Model file for the job. Use its own axes, mm. A direction names the side the tool comes from. Give positions to 0.01 mm unless a question says otherwise; leave off trailing zeros. Order: outer loops, then holes, each group sorted by start corner. A loop starts at its lowest first (then second) coordinate and runs counter-clockwise, first axis right, second up. Notation, with made-up numbers: (40.25, 44.25) - (90.25, 44.25) arc R28 cw to (90.25, 83.25) - close; hole circle Ø3 at (81.5, 77.25). An arc over 180 degrees is marked (long way). Return JSON: item names as keys, results as strings. Group by question number.
Autodesk Inventor part; units mm, degrees
ref_plane "YZ Plane" through (0, 0, 0) normal (1, 0, 0) x (0, 1, 0)
ref_plane "XZ Plane" through (0, 0, 0) normal (0, 1, 0) x (-1, 0, 0)
ref_plane "XY Plane" through (0, 0, 0) normal (0, 0, 1) x (1, 0, 0)
sketch "Sketch1" plane through (0, 0, 0) normal (0, 0, 1) x (1, 0, 0)
  circle A0 centre (157.7925, 25.2801) radius 7.5
  circle A1 centre (157.7925, 25.2801) radius 4.05
  circle A2 centre (157.7925, -42.1199) radius 7.5
  circle A3 centre (157.7925, -42.1199) radius 4.05
  line L0 (7.5, 7.5) -> (-7.5, 7.5)
  line L1 (-7.5, 7.5) -> (-7.5, -74.9)
  line L2 (-7.5, -74.9) -> (7.5, -74.9)
  line L3 (7.5, -74.9) -> (7.5, 7.5)
  line L4 (7.5, 7.5) -> (-7.5, 7.5)
  line L5 (-7.5, 7.5) -> (-7.5, -74.9)
  line L6 (-7.5, -74.9) -> (7.5, -74.9)
  line L7 (7.5, -74.9) -> (7.5, 7.5)
  circle A4 centre (157.7925, 25.2801) radius 4.05
  circle A5 centre (157.7925, 25.2801) radius 7.5
  circle A6 centre (157.7925, 25.2801) radius 4.05
  circle A7 centre (157.7925, -42.1199) radius 4.05
  circle A8 centre (157.7925, -42.1199) radius 7.5
  circle A9 centre (157.7925, -42.1199) radius 4.05
  line L8 (7.5, 7.5) -> (-7.5, 7.5)
  line L9 (-7.5, 7.5) -> (-7.5, -74.9)
  line L10 (-7.5, -74.9) -> (7.5, -74.9)
  line L11 (7.5, -74.9) -> (7.5, 7.5)
  point P0 (0, 0)
extrude "Extrusion1" add sketch "Sketch1" against normal blind 10 contours A0 | A2
sketch "Sketch2" plane through (157.7925, 25.2801, 0) normal (0, 0, 1) x (1, 0, 0)
  line L0 (7.5, 7.5) -> (-7.5, 7.5)
  line L1 (-7.5, 7.5) -> (-7.5, -74.9)
  line L2 (-7.5, -74.9) -> (7.5, -74.9)
  line L3 (7.5, -74.9) -> (7.5, 7.5)
  circle A0 centre (0, 0) radius 7.5
  circle A1 centre (0, 0) radius 4.05
  circle A2 centre (0, -67.4) radius 7.5
  circle A3 centre (0, -67.4) radius 4.05
  circle A4 centre (0, -33.7) radius 7.5
  circle A5 centre (0, -33.7) radius 5
  point P0 (-157.7925, -25.2801)
  point P1 (7.5, 0)
  point P2 (-7.5, 0)
  point P3 (-7.5, -67.4)
  point P4 (7.5, -67.4)
  dimension "d2" = 10
extrude "Extrusion2" add sketch "Sketch2" along normal blind 10 contours L3 A0 L0 | A0 L1 L0 | A0 | L3 A4 L1 A0 | A4 | L3 A2 L1 A4 | A2 | L3 L2 A2 | A2 L2 L1 | A1 | A3
fillet "Fillet1" radius 2 4 edges at (150.2925, -49.6199, 5) (165.2925, -49.6199, 5) (165.2925, 32.7801, 5) (150.2925, 32.7801, 5)
properties part number "constraining plate"
(1) Drop a flat-ended pin along its axis: pin 1 Ø1.5 at (x, y) = (155, 4) entering from -Z. Give the stop position or say it passes through.
(2) Slice it at A-A (z = -6.25). Give the cut face in (x, y).
(3) 3-axis set-ups, long thin cutter, end or side, ignore diameter. For faces 4 (the face through (158, 25, 0)), 5 (the face through (164.7, 32.2, 5.1)), 6 (the face through (152, -48, 0)): which of +Z, -Z, +X, -X, +Y, -Y reach the whole face in a straight line?
(4) Slice it at B-B (z = 4.5). Give the cut face in (x, y), and give its area (3 significant figures).
(5) Slice it at D-D (y = 3). Give the cut face in (x, z).
(6) Pull direction X, two halves, no side cores. Call faces 1 (the face through (152, 31, 0)), 2 (the face through (161.534, 23.729, -4.93)), 3 (the face through (150.292, -8, 5)): released by +X, released by -X, zero draft, split by the parting line, or undercut.
(7) Drill centre lines: L1, parallel to Y at x = 155, z = -7; L2, parallel to Y at x = 157.75, z = 9.25; L3, parallel to Y at x = 156, z = -6. Where is each one in solid material? Low to high.
Result set:
{
 "1": {"pin 1": "stops at z = 0"},
 "2": {"outline": "circle Ø15 at (157.79, -42.12); circle Ø15 at (157.79, 25.28); hole circle Ø8.1 at (157.79, -42.12); hole circle Ø8.1 at (157.79, 25.28)"},
 "3": {"face 4": "-Z", "face 5": "+Z, -Z, +X, +Y", "face 6": "-Z, -X, -Y"},
 "4": {"outline": "(150.29, -47.62) arc R2 ccw to (152.29, -49.62) - (163.29, -49.62) arc R2 ccw to (165.29, -47.62) - (165.29, 30.78) arc R2 ccw to (163.29, 32.78) - (152.29, 32.78) arc R2 ccw to (150.29, 30.78) - close; hole circle Ø10 at (157.79, -8.42)", "area": "1,150 mm²"},
 "5": {"outline": "(150.29, 0) - (165.29, 0) - (165.29, 10) - (150.29, 10) - close"},
 "6": {"face 1": "zero draft", "face 2": "undercut", "face 3": "released by -X"},
 "7": {"L1": "y = -49.08 to -45.05, -39.19 to -35.16, 18.32 to 22.35, 28.21 to 32.24", "L2": "y = -49.62 to -13.42, -3.42 to 32.78", "L3": "y = -49.4 to -45.75, -38.49 to -34.84, 18 to 21.65, 28.91 to 32.56"}
}
